```python
from build123d import *

# Parameters (mm, degrees)
SKETCH1_R                     = 20
BOSS_EXTRUDE1_DEPTH           = 22
CUT_EXTRUDE1_START            = -19
CUT_EXTRUDE1_DEPTH            = 19
CSK_FOR_M3_SFHCS1_D           = 3.6
CSK_FOR_M3_SFHCS1_CSINK_D     = 6.72
CSK_FOR_M3_SFHCS1_CSINK_ANGLE = 90
CUT_EXTRUDE2_START            = -20.001419
SKETCH7_R                     = 75
SKETCH7_R_2                   = 50
CUT_EXTRUDE2_DEPTH            = 40.002838
CUT_EXTRUDE3_REACH            = 37.833
CUT_EXTRUDE3_END_RADIUS       = 20
SKETCH8_R                     = 1.5


with BuildPart() as part:
    # Sketch1 → Boss-Extrude1 (new body)
    with BuildSketch(Plane(origin=(0, 0, 0), x_dir=(0, 0, -1), z_dir=(1, 0, 0))):
        Circle(SKETCH1_R)
    extrude(amount=BOSS_EXTRUDE1_DEPTH)

    # Sketch2 → Cut-Extrude1 (cut)
    with BuildSketch(Plane(origin=(22, 0, 0), x_dir=(0, 0, -1), z_dir=(1, 0, 0)).offset(CUT_EXTRUDE1_START)):
        with BuildLine():
            Line((-8, -18.33030278), (-8, -2.015564437))
            ThreePointArc((-8, -2.015564437), (0, 8.25), (8, -2.015564437))
            Line((8, -2.015564437), (8, -18.33030278))
            ThreePointArc((8, -18.33030278), (0, -20), (-8, -18.33030278))
        make_face()
    extrude(amount=CUT_EXTRUDE1_DEPTH, mode=Mode.SUBTRACT)

    # CSK for M3 SFHCS1 (through all)
    with Locations(Plane.ZY):
        with Locations((-12, 0), (12, 0)):
            CounterSinkHole(CSK_FOR_M3_SFHCS1_D / 2, CSK_FOR_M3_SFHCS1_CSINK_D / 2, counter_sink_angle=CSK_FOR_M3_SFHCS1_CSINK_ANGLE)

    # Sketch7 → Cut-Extrude2 (cut)
    with BuildSketch(Plane(origin=(0, 0, 0), x_dir=(1, 0, 0), z_dir=(0, 1, 0)).offset(CUT_EXTRUDE2_START)):
        with Locations((50, 0)):
            Circle(SKETCH7_R)
        with Locations((50, 0)):
            Circle(SKETCH7_R_2, mode=Mode.SUBTRACT)
    extrude(amount=CUT_EXTRUDE2_DEPTH, mode=Mode.SUBTRACT)

    # Cut-Extrude3: up to this cylinder (the profile starts inside it)
    cut_extrude3_end = Plane(origin=(9.5, 0, 0), z_dir=(-1, 0, 0)) * Cylinder(CUT_EXTRUDE3_END_RADIUS, 116.666, mode=Mode.PRIVATE)
    # Sketch8 → Cut-Extrude3 (cut, up to the surface)
    with BuildSketch(Plane.XY, mode=Mode.PRIVATE) as cut_extrude3_sk1:
        with Locations(Location((9.5, -9, 0), (0, 0, 180))):
            Circle(SKETCH8_R)
    cut_extrude3_tool1 = extrude(cut_extrude3_sk1.sketch, amount=CUT_EXTRUDE3_REACH, mode=Mode.PRIVATE) & cut_extrude3_end
    add(cut_extrude3_tool1.solids().sort_by_distance((9.5, -9, 0))[0], mode=Mode.SUBTRACT)


solid = part.part
```
The listing builds one solid part. Answer for the finished solid, in the listing's coordinates (mm). A direction names the side the tool comes from. Round coordinates to 2 decimals unless told otherwise and drop trailing zeros. Write each loop counter-clockwise with the first axis right and the second up, starting at its lowest first coordinate (ties: lowest second). Pieces come first, ordered by that corner, then holes. Notation, with made-up numbers: (48, -19) -> (65, -19) arc R7 cw to (65, -12) -> close; hole circle Ø10 at (41, -9). An arc over 180 degrees is marked (long way). Use CSV: the item, a comma, the result in double quotes. Start each with the question number.
(1) Each of these flat-tipped pins is pushed along its axis until it touches: pin 1 (3 mm diameter, centred on y = 0, z = -12, fed in from +X); pin 2 (1.5 mm diameter, centred on x = 10.5, z = -5, fed in from +Y); pin 3 (5 mm diameter, centred on x = 13.5, y = -12.5, fed in from -Z); pin 4 (5 mm diameter, centred on x = 5, y = 9.5, fed in from -Z) (3 decimals). Where does it stop, or does it pass through?
(2) Section A-A on x = 9.75 is taken. Give the vertices of the cut face in (y, z), then the cut area to 3 significant figures.
(3) Section C-C on x = 14.25 is taken. Give the vertices of the cut face in (y, z), then the cut area to 3 significant figures.
(4) Section D-D on z = 0 is taken. Give the vertices of the cut face in (x, y), then the cut area to 3 significant figures.
(5) Which of the six approach directions +Z, -Z, +X, -X, +Y, -Y give full straight-line access (tool end or side, diameter ignored) to faces 4 (the face through (12.367, 8.247, 0.21)), 5 (the face through (12, -10, -8)), 6 (the face through (9.825, -7.536, 13.196))?
(6) Consider L1, parallel to Z at x = 3.75, y = -12.5; L2, parallel to X at y = -13.5, z = 0.5; L3, parallel to X at y = -9, z = 13. Determine where each line is inside the solid, lowest interval first. Write a range as from..to.
(7) Section B-B on y = 0 is taken. Give the vertices of the cut face in (x, z), then the cut area to 3 significant figures.
(8) The mould has two halves that part along Y. Classify faces 1 (the face through (12, -10, 8)), 2 (the face through (1.39, -0.05, 10.03)), 3 (the face through (10.85, 19.83, 2.6)): released by +Y, released by -Y, zero draft, split by the parting line, or undercut.
A:
1,pin 1,"passes through"
1,pin 2,"stops at y = 19.54"
1,pin 3,"stops at z = -17.32"
1,pin 4,"stops at z = -18.735"
2,outline,"(-18.33, -8) arc R20 ccw (long way) to (-7.52, 18.53) -> (-7.52, 8) -> (-2.02, 8) arc R8.25 cw (long way) to (-2.02, -8) -> close; (-18.33, 8) -> (-10.48, 8) -> (-10.48, 17.03) arc R20 ccw to start; hole circle Ø3.6 at (0, -12); hole circle Ø3.6 at (0, 12)"
2,area,"788 mm²"
3,outline,"(-18.33, -8) arc R20 ccw (long way) to (-18.33, 8) -> (-2.02, 8) arc R8.25 cw (long way) to (-2.02, -8) -> close; hole circle Ø3.6 at (0, -12); hole circle Ø3.6 at (0, 12)"
3,area,"817 mm²"
4,outline,"(0, -20) -> (3, -20) -> (3, 8.25) -> (22, 8.25) -> (22, 20) -> (0, 20) -> close"
4,area,"343 mm²"
5,face 4,"+X"
5,face 5,"+X, -Y"
5,face 6,"+Z"
6,L1,"z = -15.61..-8, 8..15.61"
6,L2,"x = 0..3"
6,L3,"x = 1.72..8, 11..22"
7,outline,"(0.92, -9.56) -> (1.56, -10.2) -> (22, -10.2) -> (22, -8.25) -> (3, -8.25) -> (3, 8.25) -> (22, 8.25) -> (22, 10.2) -> (1.56, 10.2) -> (0.92, 9.56) arc R50 ccw to start; (1.94, -13.8) arc R50 ccw to (4.17, -20) -> (22, -20) -> (22, -13.8) -> close; (1.94, 13.8) -> (22, 13.8) -> (22, 20) -> (4.17, 20) arc R50 ccw to start"
7,area,"364 mm²"
8,face 1,"zero draft"
8,face 2,"undercut"
8,face 3,"split by the parting line"
